```python
from build123d import *

# Parameters (mm, degrees)
SCHIZZO1_W                       = 18
SCHIZZO1_H                       = 98
BASE_FLANGIA1_DEPTH              = 2
BORDO_FLANGIA1_STRIP_W           = 9.4732
BORDO_FLANGIA1_STRIP_H           = 2
BORDO_FLANGIA1_STRIP_CUT_DEPTH   = 98
BORDO_FLANGIA1_STRIP_2_W         = 9.4732
BORDO_FLANGIA1_STRIP_2_H         = 2
BORDO_FLANGIA1_STRIP_CUT_2_DEPTH = 98
BORDO_FLANGIA1_DEPTH             = 98
BORDO_FLANGIA1_BEND_DEPTH        = 98
TAGLIO_ESTRUSIONE2_DEPTH         = 111.891839195
TAGLIO_ESTRUSIONE2_DEPTH_BACK    = 111.891839195
BORDO_FLANGIA2_STRIP_W           = 9.4732
BORDO_FLANGIA2_STRIP_H           = 2
BORDO_FLANGIA2_STRIP_CUT_DEPTH   = 43
BORDO_FLANGIA2_STRIP_2_W         = 9.4732
BORDO_FLANGIA2_STRIP_2_H         = 2
BORDO_FLANGIA2_STRIP_CUT_2_DEPTH = 43
BORDO_FLANGIA2_DEPTH             = 43
BORDO_FLANGIA2_BEND_DEPTH        = 43
TAGLIO_ESTRUSIONE3_DEPTH         = 114.340195871
TAGLIO_ESTRUSIONE3_DEPTH_BACK    = 114.340195871
SCHIZZO7_R                       = 1.5
SCHIZZO8_R                       = 2.5
TAGLIO_ESTRUSIONE5_DEPTH         = 112.991071073
SCHIZZO9_R                       = 2.5
TAGLIO_ESTRUSIONE6_DEPTH         = 112.991071073
TAGLIO_ESTRUSIONE7_DEPTH         = 114.340195871
TAGLIO_ESTRUSIONE7_DEPTH_BACK    = 114.340195871
SCHIZZO10_RX                     = 6
SCHIZZO10_RY                     = 3
SCHIZZO11_W                      = 20
SCHIZZO11_H                      = 3.5
TAGLIO_ESTRUSIONE8_DEPTH         = 9
BORDO_FLANGIA4_START             = -60
BORDO_FLANGIA4_DEPTH             = 22
BORDO_FLANGIA4_2_DEPTH           = 1
BORDO_FLANGIA4_START_2           = -39
BORDO_FLANGIA4_3_DEPTH           = 1
BORDO_FLANGIA4_START_3           = -59
BORDO_FLANGIA4_4_DEPTH           = 20
SCHIZZO13_R                      = 2.5
TAGLIO_ESTRUSIONE9_DEPTH         = 9


# Read off the part's stored shape, not the designer's step: Bordo-Flangia4
# Sheet-metal steps are written as plain solids
with BuildPart() as part:
    # Schizzo1 → Base-Flangia1 (new body)
    with BuildSketch(Plane(origin=(0, 0, 0), x_dir=(1, 0, 0), z_dir=(0, 1, 0))):
        with Locations((9, 49)):
            Rectangle(SCHIZZO1_W, SCHIZZO1_H)
    extrude(amount=BASE_FLANGIA1_DEPTH)

    # Bordo-Flangia1 strip (across the edge) → Bordo-Flangia1 strip cut (cut)
    with BuildSketch(Plane(origin=(0, 2, -98), x_dir=(1, 0, 0), z_dir=(0, 0, 1))):
        with Locations((-4, -1)):
            Rectangle(BORDO_FLANGIA1_STRIP_W, BORDO_FLANGIA1_STRIP_H)
    extrude(amount=BORDO_FLANGIA1_STRIP_CUT_DEPTH, mode=Mode.SUBTRACT)

    # Bordo-Flangia1 strip 2 (across the edge) → Bordo-Flangia1 strip cut 2 (cut)
    with BuildSketch(Plane(origin=(18, 2, 0), x_dir=(-1, 0, 0), z_dir=(0, 0, -1))):
        with Locations((-4, -1)):
            Rectangle(BORDO_FLANGIA1_STRIP_2_W, BORDO_FLANGIA1_STRIP_2_H)
    extrude(amount=BORDO_FLANGIA1_STRIP_CUT_2_DEPTH, mode=Mode.SUBTRACT)

    # Bordo-Flangia1 section (across the edge) → Bordo-Flangia1 (add)
    with BuildSketch(Plane(origin=(0, 2, -98), x_dir=(1, 0, 0), z_dir=(0, 0, 1))):
        with BuildLine():
            Line((-2, 0.7366), (-2, 45))
            Line((-2, 45), (0, 45))
            Line((0, 45), (0, 0.7366))
            ThreePointArc((0, 0.7366), (0.215745145, 0.215745145), (0.7366, 0))
            Line((0.7366, 0), (0.7366, -2))
            ThreePointArc((0.7366, -2), (-1.198468417, -1.198468417), (-2, 0.7366))
        make_face()
    extrude(amount=BORDO_FLANGIA1_DEPTH)

    # Bordo-Flangia1 section 2 (across the edge) → Bordo-Flangia1 bend (add)
    with BuildSketch(Plane(origin=(18, 2, 0), x_dir=(-1, 0, 0), z_dir=(0, 0, -1))):
        with BuildLine():
            Line((-2, 0.7366), (-2, 45))
            Line((-2, 45), (0, 45))
            Line((0, 45), (0, 0.7366))
            ThreePointArc((0, 0.7366), (0.215745145, 0.215745145), (0.7366, 0))
            Line((0.7366, 0), (0.7366, -2))
            ThreePointArc((0.7366, -2), (-1.198468417, -1.198468417), (-2, 0.7366))
        make_face()
    extrude(amount=BORDO_FLANGIA1_BEND_DEPTH)

    # Schizzo4 → Taglio-Estrusione2 (cut, two sides: drawn at the far end of the back side and taken through both)
    with BuildSketch(Plane.ZY.offset(2).offset(-TAGLIO_ESTRUSIONE2_DEPTH_BACK)):
        Polygon((-98, 47), (-98, 21.7366), (-70.5, 34), (-70.5, 47), align=None)
        Polygon((-27.5, 34), (0, 21.7366), (0, 47), (-27.5, 47), align=None)
    extrude(amount=TAGLIO_ESTRUSIONE2_DEPTH + TAGLIO_ESTRUSIONE2_DEPTH_BACK, mode=Mode.SUBTRACT)

    # Bordo-Flangia2 strip (across the edge) → Bordo-Flangia2 strip cut (cut)
    with BuildSketch(Plane(origin=(20, 47, -70.5), x_dir=(0, -1, 0), z_dir=(0, 0, 1))):
        with Locations((-4, -1)):
            Rectangle(BORDO_FLANGIA2_STRIP_W, BORDO_FLANGIA2_STRIP_H)
    extrude(amount=BORDO_FLANGIA2_STRIP_CUT_DEPTH, mode=Mode.SUBTRACT)

    # Bordo-Flangia2 strip 2 (across the edge) → Bordo-Flangia2 strip cut 2 (cut)
    with BuildSketch(Plane(origin=(-2, 47, -27.5), x_dir=(0, -1, 0), z_dir=(0, 0, -1))):
        with Locations((-4, -1)):
            Rectangle(BORDO_FLANGIA2_STRIP_2_W, BORDO_FLANGIA2_STRIP_2_H)
    extrude(amount=BORDO_FLANGIA2_STRIP_CUT_2_DEPTH, mode=Mode.SUBTRACT)

    # Bordo-Flangia2 section (across the edge) → Bordo-Flangia2 (add)
    with BuildSketch(Plane(origin=(20, 47, -70.5), x_dir=(0, -1, 0), z_dir=(0, 0, 1))):
        with BuildLine():
            Line((-2, 0.7366), (-2, 7))
            Line((-2, 7), (0, 7))
            Line((0, 7), (0, 0.7366))
            ThreePointArc((0, 0.7366), (0.215745145, 0.215745145), (0.7366, 0))
            Line((0.7366, 0), (0.7366, -2))
            ThreePointArc((0.7366, -2), (-1.198468417, -1.198468417), (-2, 0.7366))
        make_face()
    extrude(amount=BORDO_FLANGIA2_DEPTH)

    # Bordo-Flangia2 section 2 (across the edge) → Bordo-Flangia2 bend (add)
    with BuildSketch(Plane(origin=(-2, 47, -27.5), x_dir=(0, -1, 0), z_dir=(0, 0, -1))):
        with BuildLine():
            Line((-2, 0.7366), (-2, 7))
            Line((-2, 7), (0, 7))
            Line((0, 7), (0, 0.7366))
            ThreePointArc((0, 0.7366), (0.215745145, 0.215745145), (0.7366, 0))
            Line((0.7366, 0), (0.7366, -2))
            ThreePointArc((0.7366, -2), (-1.198468417, -1.198468417), (-2, 0.7366))
        make_face()
    extrude(amount=BORDO_FLANGIA2_BEND_DEPTH)

    # Schizzo7 → Taglio-Estrusione3 (cut, two sides: drawn at the far end of the back side and taken through both)
    with BuildSketch(Plane.ZY.offset(2).offset(-TAGLIO_ESTRUSIONE3_DEPTH_BACK)):
        with Locations(Location((-66.5, 38.2634, 0), (0, 0, 270))):
            Circle(SCHIZZO7_R)
        with Locations(Location((-31.5, 38.2634, 0), (0, 0, 270))):
            Circle(SCHIZZO7_R)
        with Locations(Location((-92, 10.7366, 0), (0, 0, 270))):
            Circle(SCHIZZO7_R)
        with Locations(Location((-6, 10.7366, 0), (0, 0, 270))):
            Circle(SCHIZZO7_R)
        with Locations(Location((-76, 10.7366, 0), (0, 0, 270))):
            Circle(SCHIZZO7_R)
        with Locations(Location((-22, 10.7366, 0), (0, 0, 270))):
            Circle(SCHIZZO7_R)
    extrude(amount=TAGLIO_ESTRUSIONE3_DEPTH + TAGLIO_ESTRUSIONE3_DEPTH_BACK, mode=Mode.SUBTRACT)

    # Schizzo8 → Taglio-Estrusione5 (cut, through all)
    with BuildSketch(Plane.XZ.offset(-47)):
        with Locations(Location((23.5, -31.5, 0), (0, 0, 270))):
            Circle(SCHIZZO8_R)
        with Locations(Location((23.5, -66.5, 0), (0, 0, 270))):
            Circle(SCHIZZO8_R)
    extrude(amount=-TAGLIO_ESTRUSIONE5_DEPTH, mode=Mode.SUBTRACT)

    # Schizzo9 → Taglio-Estrusione6 (cut, through all)
    with BuildSketch(Plane.XZ.offset(-47)):
        with Locations(Location((-5.5, -31.5, 0), (0, 0, 270))):
            Circle(SCHIZZO9_R)
        with Locations(Location((-5.5, -66.5, 0), (0, 0, 270))):
            Circle(SCHIZZO9_R)
    extrude(amount=-TAGLIO_ESTRUSIONE6_DEPTH, mode=Mode.SUBTRACT)

    # Schizzo10 → Taglio-Estrusione7 (cut, two sides: drawn at the far end of the back side and taken through both)
    with BuildSketch(Plane.ZY.offset(2).offset(-TAGLIO_ESTRUSIONE7_DEPTH_BACK)):
        with Locations(Location((-59, 10.7366), (0, 0, -90))):
            Ellipse(SCHIZZO10_RX, SCHIZZO10_RY)
        with Locations(Location((-39, 10.7366), (0, 0, 90))):
            Ellipse(SCHIZZO10_RX, SCHIZZO10_RY)
    extrude(amount=TAGLIO_ESTRUSIONE7_DEPTH + TAGLIO_ESTRUSIONE7_DEPTH_BACK, mode=Mode.SUBTRACT)

    # Schizzo11 → Taglio-Estrusione8 (cut)
    with BuildSketch(Plane.ZY.offset(2)):
        with Locations((-49, 44.5134)):
            Rectangle(SCHIZZO11_W, SCHIZZO11_H)
    extrude(amount=-TAGLIO_ESTRUSIONE8_DEPTH, mode=Mode.SUBTRACT)

    # Bordo-Flangia4 outline → Bordo-Flangia4 (cut)
    with BuildSketch(Plane.XY.offset(BORDO_FLANGIA4_START)):
        with BuildLine():
            Line((0, 42.7634), (-2, 42.7634))
            Line((-2, 42.7634), (-2, 42.662402398))
            ThreePointArc((-2, 42.662402398), (-0.556604688, 41.681067209), (0, 40.0268))
            Line((0, 40.0268), (0, 42.7634))
        make_face()
    extrude(amount=BORDO_FLANGIA4_DEPTH, mode=Mode.SUBTRACT)

    # Bordo-Flangia4 2 outline → Bordo-Flangia4 2 (cut)
    with BuildSketch(Plane.XY.offset(BORDO_FLANGIA4_START)):
        with BuildLine():
            ThreePointArc((0, 40.0268), (-0.556604688, 41.681067209), (-2, 42.662402398))
            Line((-2, 42.662402398), (-2, 39.0268))
            Line((-2, 39.0268), (0, 39.0268))
            Line((0, 39.0268), (0, 40.0268))
        make_face()
    extrude(amount=BORDO_FLANGIA4_2_DEPTH, mode=Mode.SUBTRACT)

    # Bordo-Flangia4 3 outline → Bordo-Flangia4 3 (cut)
    with BuildSketch(Plane.XY.offset(BORDO_FLANGIA4_START_2)):
        with BuildLine():
            ThreePointArc((0, 40.0268), (-0.556604688, 41.681067209), (-2, 42.662402398))
            Line((-2, 42.662402398), (-2, 39.0268))
            Line((-2, 39.0268), (0, 39.0268))
            Line((0, 39.0268), (0, 40.0268))
        make_face()
    extrude(amount=BORDO_FLANGIA4_3_DEPTH, mode=Mode.SUBTRACT)

    # Bordo-Flangia4 4 outline → Bordo-Flangia4 4 (add)
    with BuildSketch(Plane.XY.offset(BORDO_FLANGIA4_START_3)):
        with BuildLine():
            Line((-2, 40.0268), (-2, 42.662402398))
            ThreePointArc((-2, 42.662402398), (-2.364854094, 42.738033029), (-2.7366, 42.7634))
            Line((-2.7366, 42.7634), (-8, 42.7634))
            Line((-8, 42.7634), (-8, 40.7634))
            Line((-8, 40.7634), (-2.7366, 40.7634))
            ThreePointArc((-2.7366, 40.7634), (-2.215745145, 40.547654855), (-2, 40.0268))
        make_face()
    extrude(amount=BORDO_FLANGIA4_4_DEPTH)

    # Schizzo13 → Taglio-Estrusione9 (cut)
    with BuildSketch(Plane.XZ):
        with Locations(Location((9, -49, 0), (0, 0, 270))):
            Circle(SCHIZZO13_R)
    extrude(amount=-TAGLIO_ESTRUSIONE9_DEPTH, mode=Mode.SUBTRACT)


solid = part.part
```
Source: CAD feature listing. Evaluate the final solid. Frame: model axes, mm. A direction names the side the tool comes from. Round coordinates to 2 decimals unless told otherwise and drop trailing zeros. Loops run counter-clockwise (first coordinate to the right, second up) from the corner with the lowest first, then second, coordinate; pieces in that order, holes last.
1. Mould query, pull axis X, two halves, no side actions, for faces 1 (the flat face through (-6, 47, -49)), 2 (the flat face through (-9, 48, -49)), 3 (the cylindrical face through (25.61, 47.99, -67.84)). Classes: released by +X, released by -X, zero draft, split by the parting line, or undercut.
2. Section query A-A on x = 23.5. Output: boundary loops of the cut face in (y, z), and give its area (3 significant figures).
3. Section query C-C on y = 29. Output: boundary loops of the cut face in (x, z), and give its area (3 significant figures).
4. Ray query, L1, parallel to X at y = 5, z = -31; L2, parallel to X at y = 48.3, z = -31.5; L3, parallel to Y at x = -1.4, z = -31.5. Return the intervals inside material, ascending.
5. Section query B-B on z = -49. Give the number of separate pieces and of enclosed holes in the cut face, and give its area (3 significant figures).
6. Access query for faces 4 (the flat face through (-1.5, 43.7, -70.5)), 5 (the flat face through (24, 47, -49)), 6 (the flat face through (-1, 44, -59)). Directions: +Z, -Z, +X, -X, +Y, -Y. A direction counts if a zero-diameter tool reaches every point of the face in a straight line with its end or side. Return the directions, or none.
7. Contact query for flat-ended pins moving along their axis: pin 1 (8 mm diameter, centred on x = 9, y = 7, fed in from +Z); pin 2 (4 mm diameter, centred on x = 1, z = -54.5, fed in from -Y); pin 3 (5 mm diameter, centred on x = 11.5, z = -80, fed in from +Y); pin 4 (1.6 mm diameter, centred on x = -0.5, y = 44.5, fed in from +Z). Output: stop coordinate, or through.
Answers below:
1. face 1: zero draft
1. face 2: released by -X
1. face 3: undercut
2. outline: (47, -70.5) - (49, -70.5) - (49, -69) - (47, -69) - close; (47, -64) - (49, -64) - (49, -34) - (47, -34) - close; (47, -29) - (49, -29) - (49, -27.5) - (47, -27.5) - close
2. area: 66.0 mm2
3. outline: (-2, -81.71) - (0, -81.71) - (0, -16.29) - (-2, -16.29) - close; (18, -81.71) - (20, -81.71) - (20, -16.29) - (18, -16.29) - close
3. area: 262 mm2
4. L1: x = -2 to 0, 18 to 20
4. L2: x = -9 to -8, -3 to -0.91, 18.91 to 21, 26 to 27
4. L3: y = 1.03 to 36.76, 39.76 to 48.65
5. separate pieces: 3
5. enclosed holes: 0
5. area: 248 mm2
6. face 4: -Z, +X, -X, +Y
6. face 5: +Z, -Z, +X, -Y
6. face 6: -X
7. pin 1: passes through
7. pin 2: stops at y = 0
7. pin 3: stops at y = 2
7. pin 4: stops at z = -27.5
